Source: CAD feature listing. Evaluate the final solid. Frame: model axes, mm. Round coordinates to 2 decimals unless told otherwise and drop trailing zeros. Write each loop counter-clockwise with the first axis right and the second up, starting at its lowest first coordinate (ties: lowest second). Pieces come first, ordered by that corner, then holes. Notation, with made-up numbers: (84, -26) - (136, -26) arc R18 cw to (136, -22) - close; hole circle Ø7 at (28, 23). An arc over 180 degrees is marked (long way). Write item = value, one per line. Start each with the question number.
```python
from build123d import *

# Parameters (mm, degrees)
BOSS_EXTRUDE1_DEPTH = 1
FILLET1_R           = 10
SKETCH2_R           = 4.5
CUT_EXTRUDE1_DEPTH  = 10


with BuildPart() as part:
    # Sketch1 → Boss-Extrude1 (new body)
    with BuildSketch(Plane.XY):
        with BuildLine():
            Line((0, 0), (70, 0))
            ThreePointArc((70, 0), (79.920098672, 8.738396919), (72.50304541, 19.681671533))
            ThreePointArc((72.50304541, 19.681671533), (38.890872965, 38.890872965), (19.681671533, 72.50304541))
            ThreePointArc((19.681671533, 72.50304541), (8.738396919, 79.920098672), (0, 70))
            Line((0, 70), (0, 0))
        make_face()
    extrude(amount=BOSS_EXTRUDE1_DEPTH)

    # Fillet1
    fillet1_edges = [part.edges().sort_by_distance(p)[0] for p in [
        (0, 0, 0.5),
    ]]
    fillet(fillet1_edges, radius=FILLET1_R)

    # Sketch2 → Cut-Extrude1 (cut)
    with BuildSketch(Plane.XY.offset(1)):
        with Locations((10, 10)):
            Circle(SKETCH2_R)
        with Locations((70, 10)):
            Circle(SKETCH2_R)
        with Locations((10, 70)):
            Circle(SKETCH2_R)
    extrude(amount=-CUT_EXTRUDE1_DEPTH, mode=Mode.SUBTRACT)


solid = part.part
```
(1) Pull-direction query (X, two-part tool) for faces 1 (the cylindrical face through (3.01, 2.85, 0.51)), 2 (the flat face through (31, 32, 0)), 3 (the cylindrical face through (9.41, 74.46, 0.51)), 4 (the cylindrical face through (79.893, 8.538, 0.493)); classes: +X half, -X half, draft (parallel to the pull), parting line (faces both ways), or undercut.
(2) Contact query for a flat-ended pin moving along its axis: P1, Ø1, axis at x = 25, y = 55.5, coming from the -Z side. Output: stop coordinate, or through.
(3) Section A-A (z = 0.7). Return the cut outline in (x, y).
(4) Ray query, L1, parallel to Y at x = 10, z = 0.8; L2, parallel to Y at x = 70, z = 0.7; L3, parallel to X at y = 13, z = 0.5. Return the intervals inside material, ascending. Write a range as from..to.
(5) Section C-C (x = 67). Return the cut outline in (y, z), plus the area to 3 significant figures.
(6) Section D-D (y = 64). Return the cut outline in (x, z).
(7) Section B-B (x = 8). Return the cut outline in (y, z).
Solution:
q1.face_1 = -X half
q1.face_2 = draft
q1.face_3 = undercut
q1.face_4 = +X half
q2.P1 = 0
q3.outline = (0, 10) arc R10 ccw to (10, 0) - (70, 0) arc R10 ccw to (72.5, 19.68) arc R73.58 cw to (19.68, 72.5) arc R10 ccw to (0, 70) - close; hole circle Ø9 at (10, 10); hole circle Ø9 at (10, 70); hole circle Ø9 at (70, 10)
q4.L1 = 0..5.5, 14.5..65.5, 74.5..80
q4.L2 = 0..5.5, 14.5..20.38
q4.L3 = 0..6.65, 13.35..66.65, 73.35..79.54
q5.outline = (0, 0) - (6.65, 0) - (6.65, 1) - (0, 1) - close; (13.35, 0) - (21.34, 0) - (21.34, 1) - (13.35, 1) - close
q5.area = 14.6 mm^2
q6.outline = (0, 0) - (22.44, 0) - (22.44, 1) - (0, 1) - close
q7.outline = (0.2, 0) - (5.97, 0) - (5.97, 1) - (0.2, 1) - close; (14.03, 0) - (65.97, 0) - (65.97, 1) - (14.03, 1) - close; (74.03, 0) - (79.8, 0) - (79.8, 1) - (74.03, 1) - close
